```python
from build123d import *

# Parameters (mm, degrees)
SKETCH2_W           = 170
SKETCH2_H           = 85
BOSS_EXTRUDE1_DEPTH = 2
SKETCH3_W           = 12
SKETCH3_H           = 15
CUT_EXTRUDE1_DEPTH  = 106.73546699
SKETCH6_W           = 170
SKETCH6_H           = 3
BOSS_EXTRUDE2_DEPTH = 100
SKETCH7_W           = 170
SKETCH7_H           = 2.5
BOSS_EXTRUDE3_DEPTH = 15
SKETCH8_W           = 170
SKETCH8_H           = 2.5
BOSS_EXTRUDE4_DEPTH = 15
SKETCH9_R           = 1.7
CUT_EXTRUDE3_DEPTH  = 151.557944579
SKETCH11_R          = 1.7
CUT_EXTRUDE4_DEPTH  = 151.557944579


with BuildPart() as part:
    # Sketch2 → Boss-Extrude1 (new body)
    with BuildSketch(Plane(origin=(0, 0, 0), x_dir=(1, 0, 0), z_dir=(0, 1, 0))):
        with Locations((10.400843882, -3.048523207)):
            Rectangle(SKETCH2_W, SKETCH2_H)
    extrude(amount=BOSS_EXTRUDE1_DEPTH)

    # Sketch3 → Cut-Extrude1 (cut, through all)
    with BuildSketch(Plane(origin=(0, 2, 0), x_dir=(1, 0, 0), z_dir=(0, 1, 0))):
        with Locations((-35.599156118, 28.951476793)):
            Rectangle(SKETCH3_W, SKETCH3_H)
    extrude(amount=-CUT_EXTRUDE1_DEPTH, mode=Mode.SUBTRACT)

    # Sketch6 → Boss-Extrude2 (add)
    with BuildSketch(Plane.XZ):
        with Locations((10.400843882, -37.951476793)):
            Rectangle(SKETCH6_W, SKETCH6_H)
        with Locations((10.400843882, 44.048523207)):
            Rectangle(SKETCH6_W, SKETCH6_H)
    extrude(amount=BOSS_EXTRUDE2_DEPTH)

    # Sketch7 → Boss-Extrude3 (add)
    with BuildSketch(Plane(origin=(0, 0, -39.451476793), x_dir=(-1, 0, 0), z_dir=(0, 0, -1))):
        with Locations((-10.400843882, -98.75)):
            Rectangle(SKETCH7_W, SKETCH7_H)
    extrude(amount=BOSS_EXTRUDE3_DEPTH)

    # Sketch8 → Boss-Extrude4 (add)
    with BuildSketch(Plane.XY.offset(45.548523207)):
        with Locations((10.400843882, -98.75)):
            Rectangle(SKETCH8_W, SKETCH8_H)
    extrude(amount=BOSS_EXTRUDE4_DEPTH)

    # Sketch9 → Cut-Extrude3 (cut, through all)
    with BuildSketch(Plane(origin=(0, -97.5, 0), x_dir=(1, 0, 0), z_dir=(0, 1, 0))):
        with Locations(Location((5.400843882, -53.048523207, 0), (0, 0, 270))):
            Circle(SKETCH9_R)
        with Locations(Location((15.400843882, -53.048523207, 0), (0, 0, 270))):
            Circle(SKETCH9_R)
    extrude(amount=-CUT_EXTRUDE3_DEPTH, mode=Mode.SUBTRACT)

    # Sketch11 → Cut-Extrude4 (cut, through all)
    with BuildSketch(Plane(origin=(0, -97.5, 0), x_dir=(1, 0, 0), z_dir=(0, 1, 0))):
        with Locations(Location((5.400843882, 46.951476793, 0), (0, 0, 270))):
            Circle(SKETCH11_R)
        with Locations(Location((15.400843882, 46.951476793, 0), (0, 0, 270))):
            Circle(SKETCH11_R)
    extrude(amount=-CUT_EXTRUDE4_DEPTH, mode=Mode.SUBTRACT)


solid = part.part
```
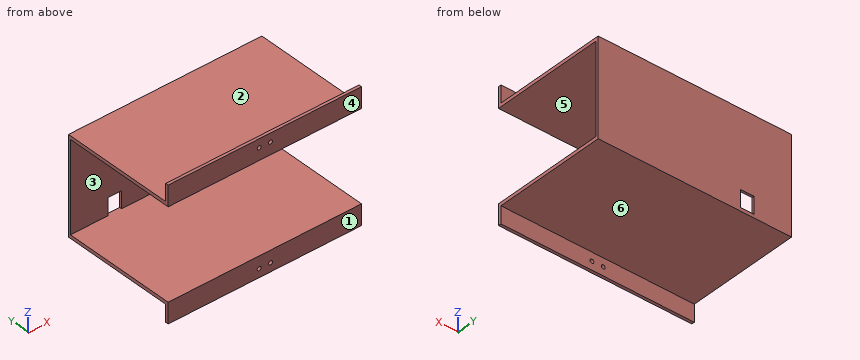
Can you work these out from the model? Positions are in its coordinate system, mm. Face numbers are marked on the shaded views. A direction names the side the tool comes from. Coordinates: 2 decimals unless noted, no trailing zeros. Order: outer loops, then holes, each group sorted by start corner. A loop starts at its lowest first (then second) coordinate and runs counter-clockwise, first axis right, second up. Notation, with made-up numbers: (-21.75, 63.5) - (13.25, 63.5) arc R31 ccw to (13.25, 89.5) - close; hole circle Ø9 at (74.25, 76). An arc over 180 degrees is marked (long way). Answer in a Markdown table with one row per item.
1. For the marked faces 1, 2 and 3, which set-ups out of +Z, -Z, +X, -X, +Y, -Y let a thin tool reach every point of the face, with its end or its side?
Reply:
| item | result |
|---|---|
| face 1 | +Z, -Z, +X, -X, -Y |
| face 2 | +Z, +X, -X, +Y |
| face 3 | +X, -X, -Y |
2. Suppose I cut it at C-C (z = 8). Please give me the cut outline in (x, y).
Reply:
| item | result |
|---|---|
| outline | (-74.6, 0) - (95.4, 0) - (95.4, 2) - (-74.6, 2) - close |
3. For pin 1 (6 mm diameter, centred on y = -23, z = -35, fed in from -X); pin 2 (16.5 mm diameter, centred on x = -25, z = 55, fed in from +Y); pin 3 (10 mm diameter, centred on x = 13, z = 27, fed in from -Y); pin 4 (1.6 mm diameter, centred on x = -32.5, y = 1.5, fed in from -Z), each with a flat end and sliding along its axis, tell me the tip position at first contact or that it passes through.
Reply:
| item | result |
|---|---|
| pin 1 | stops at x = -74.6 |
| pin 2 | stops at y = -97.5 |
| pin 3 | stops at y = 0 |
| pin 4 | stops at z = -39.45 |
4. Suppose I cut it at B-B (x = 53). Please give me the cut outline in (y, z).
Reply:
| item | result |
|---|---|
| outline | (-100, -54.45) - (-97.5, -54.45) - (-97.5, -39.45) - (2, -39.45) - (2, 45.55) - (-97.5, 45.55) - (-97.5, 60.55) - (-100, 60.55) - (-100, 42.55) - (0, 42.55) - (0, -36.45) - (-100, -36.45) - close |
5. If I drill on line 1 along Z through (x, y) = (-48, -67.5); line 2 along Y through (x, z) = (41.5, -35); line 3 along Y through (x, z) = (75.5, -40), over which ranges is the centre line in solid material (lowest first)?
Reply:
| item | result |
|---|---|
| line 1 | z = -39.45 to -36.45, 42.55 to 45.55 |
| line 2 | y = 0 to 2 |
| line 3 | y = -100 to -97.5 |
6. Suppose I cut it at A-A (y = -16.5). Please give me the cut outline in (x, z).
Reply:
| item | result |
|---|---|
| outline | (-74.6, -39.45) - (95.4, -39.45) - (95.4, -36.45) - (-74.6, -36.45) - close; (-74.6, 42.55) - (95.4, 42.55) - (95.4, 45.55) - (-74.6, 45.55) - close |
7. If we mould it in two halves opening along Z, with no side actions, what happens to the marked faces 4, 5 and 6? For each: pulls with the +Z half, pulls with the -Z half, needs draft (parallel to the pull), parting line crosses it, or undercut.
Reply:
| item | result |
|---|---|
| face 4 | needs draft |
| face 5 | undercut |
| face 6 | pulls with the -Z half |
